from build123d import *

# Parameters (mm, degrees)
F1_DEPTH = 25.4
F2_W     = 13.004002
F2_H     = 18.828773
F3_DEPTH = 6.35


with BuildPart() as f1:
    # F0 (on Top) → F1 (new body)
    with BuildSketch(Plane.XY):
        Polygon((-49.004722, 32.224186), (-49.004722, -32.224186), (49.004722, -32.224186), (49.004722, 32.224186), (25.007728, 32.224186), (-25.007728, 32.224186), align=None)
    extrude(amount=F1_DEPTH)

    # F2 (on face) → F3 (cut)
    with BuildSketch(Plane.XY.offset(25.4)):
        with Locations((-28.497411, -0.615601)):
            Rectangle(F2_W, F2_H)
    extrude(amount=-F3_DEPTH, mode=Mode.SUBTRACT)


solid = f1.part
The listing builds one solid part. Answer for the finished solid, in the listing's coordinates (mm). A direction names the side the tool comes from. Give positions to 0.01 mm unless a question says otherwise; leave off trailing zeros. Write each loop counter-clockwise with the first axis right and the second up, starting at its lowest first coordinate (ties: lowest second). Pieces come first, ordered by that corner, then holes.
1) For a pull along Y with two mould halves and no side action, classify faces 1 (the face through (1, 32.224, 13)), 2 (the face through (-1, 0, 0)), 3 (the face through (-1, -32.224, 13)), 4 (the face through (-34.999, -1, 22)) as pulls with the +Y half, pulls with the -Y half, needs draft (parallel to the pull), parting line crosses it, or undercut.
2) A tool of negligible diameter and unlimited length cuts with its end or side. For faces 5 (the face through (-29, 8.799, 22)), 6 (the face through (-49.005, 0, 13)), from which of +Z, -Z, +X, -X, +Y, -Y can it reach the whole face along a straight path? Write none if from no direction.
3) Section B-B (y = -4) is taken. Write down the section's boundary in (x, z).
4) Find the intervals of material crossed by L1, parallel to X at y = -9.5, z = 19.5, in increasing order.
5) Given P1, Ø6.5, axis at x = -29.5, y = 2, coming from the +Z side, flat-ended and moving along its own axis, determine where the tip first touches the part or whether it passes through.
6) Section A-A (z = 23.5) is taken. Write down the section's boundary in (x, y), and give its area (3 significant figures).
Response:
1. face 1: pulls with the +Y half
1. face 2: needs draft
1. face 3: pulls with the -Y half
1. face 4: undercut
2. face 5: +Z
2. face 6: +Z, -Z, -X, +Y, -Y
3. outline: (-49, 0) - (49, 0) - (49, 25.4) - (-22, 25.4) - (-22, 19.05) - (-35, 19.05) - (-35, 25.4) - (-49, 25.4) - close
4. L1: x = -49 to -35, -22 to 49
5. P1: stops at z = 19.05
6. outline: (-49, -32.22) - (49, -32.22) - (49, 32.22) - (-49, 32.22) - close; hole (-35, -10.03) - (-22, -10.03) - (-22, 8.8) - (-35, 8.8) - close
6. area: 6,070 mm2
